The figure shows three views and two pictorial views of one solid part (mm, origin at its lowest corner). Answer the questions. A direction names the side the tool comes from. Give positions to 0.01 mm unless a question says otherwise; leave off trailing zeros. Order: outer loops, then holes, each group sorted by start corner. A loop starts at its lowest first (then second) coordinate and runs counter-clockwise, first axis right, second up. Notation, with made-up numbers: M 13,10.5 L 53,10.5 A29 ccw 53,47.5 Z; hole C 27,86 d10. An arc over 180 degrees is marked long. Answer as a JSON object with one key per item and string values. Group by question number.
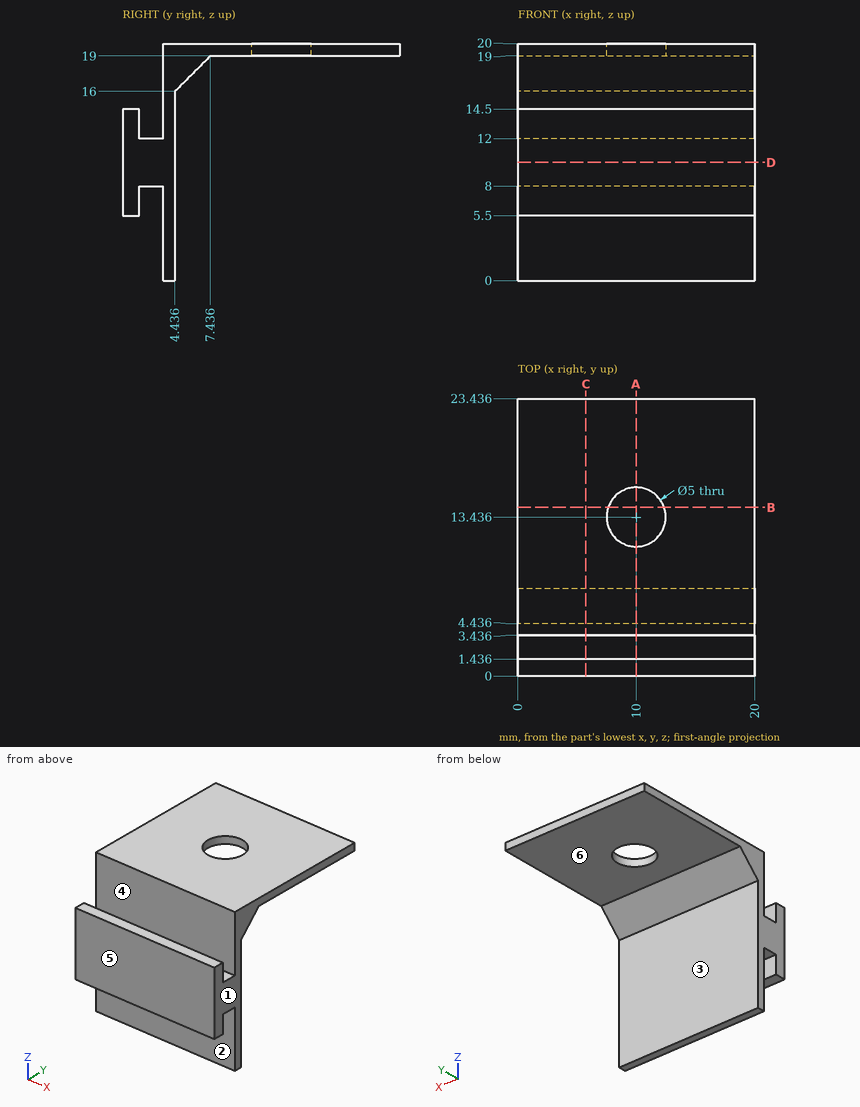
Item 1: Section A-A (x = 10) is taken. Determine the outline of the cut face in (y, z), and give its area (3 significant figures).
Item 2: Section C-C (x = 5.75) is taken. Determine the outline of the cut face in (y, z).
Item 3: A tool of negligible diameter and unlimited length cuts with its end or side. For the marked faces 5 and 6, from which of +Z, -Z, +X, -X, +Y, -Y can it reach the whole face along a straight path? Write none if from no direction.
Item 4: Determine the mould class of the marked faces 1, 2, 3 and 4 for opening direction Y: released by +Y, released by -Y, zero draft, split by the parting line, or undercut.
Item 5: Flat-ended cylindrical pins translate along their axes: P1, Ø1.6, axis at x = 6.5, y = 2.5, coming from the +Z side; P2, Ø1.6, axis at x = 12, y = 0.5, coming from the +Z side; P3, Ø3, axis at x = 14.5, z = 13, coming from the +Y side. Find the tip coordinate at first contact, or state that the pin passes through.
Item 6: Section B-B (y = 14.25) is taken. Determine the outline of the cut face in (x, z), and give its area (3 significant figures).
Item 7: Section D-D (z = 10) is taken. Determine the outline of the cut face in (x, y), and give its area (3 significant figures).
Item 8: Consider probe 1 along Y at (x, z) = (10, 19.25); probe 2 along Y at (x, z) = (17.75, 6.75); probe 3 along Y at (x, z) = (6.75, 9.75). Determine where each line is inside the solid, lowest interval first. Write a range as from..to.
Values found:
{
 "1": {"outline": "M 0,5.5 L 1.44,5.5 L 1.44,8 L 3.44,8 L 3.44,0 L 4.44,0 L 4.44,16 L 7.44,19 L 10.94,19 L 10.94,20 L 3.44,20 L 3.44,12 L 1.44,12 L 1.44,14.5 L 0,14.5 Z; M 15.94,19 L 23.44,19 L 23.44,20 L 15.94,20 Z", "area": "59.4 mm^2"},
 "2": {"outline": "M 0,5.5 L 1.44,5.5 L 1.44,8 L 3.44,8 L 3.44,0 L 4.44,0 L 4.44,16 L 7.44,19 L 23.44,19 L 23.44,20 L 3.44,20 L 3.44,12 L 1.44,12 L 1.44,14.5 L 0,14.5 Z"},
 "3": {"face 5": "+Z, -Z, +X, -X, -Y", "face 6": "-Z, +X, -X, +Y"},
 "4": {"face 1": "zero draft", "face 2": "undercut", "face 3": "released by +Y", "face 4": "undercut"},
 "5": {"P1": "stops at z = 12", "P2": "stops at z = 14.5", "P3": "stops at y = 4.44"},
 "6": {"outline": "M 0,19 L 7.64,19 L 7.64,20 L 0,20 Z; M 12.36,19 L 20,19 L 20,20 L 12.36,20 Z", "area": "15.3 mm^2"},
 "7": {"outline": "M 0,0 L 20,0 L 20,4.44 L 0,4.44 Z", "area": "88.7 mm^2"},
 "8": {"probe 1": "y = 3.44..10.94, 15.94..23.44", "probe 2": "y = 0..1.44, 3.44..4.44", "probe 3": "y = 0..4.44"}
}
